Source: CAD feature listing. Evaluate the final solid. Frame: model axes, mm. A direction names the side the tool comes from. Give positions to 0.01 mm unless a question says otherwise; leave off trailing zeros. Order: outer loops, then holes, each group sorted by start corner. A loop starts at its lowest first (then second) coordinate and runs counter-clockwise, first axis right, second up. Notation, with made-up numbers: M 19,76 L 54,76 A28 cw 54,115 Z; hole C 48.25,83.5 d1. An arc over 180 degrees is marked long. Return JSON: item names as keys, results as strings.
from build123d import *

# Parameters (mm, degrees)
SKETCH_1_W          = 25
SKETCH_1_H          = 24
EXTRUDE_1_DEPTH     = 25
SKETCH_2_W          = 25
SKETCH_2_H          = 14.5
CUT_EXTRUDE_1_DEPTH = 5
SKETCH_3_R          = 1.5
CUT_EXTRUDE_2_DEPTH = 31.417922349
CUT_EXTRUDE_3_DEPTH = 37.84087404
SKETCH_6_R          = 3.5
CUT_EXTRUDE_4_DEPTH = 13
SKETCH_7_R          = 3.5
CUT_EXTRUDE_5_DEPTH = 7
SKETCH_8_R          = 1.25
CUT_EXTRUDE_6_DEPTH = 37.84087404


with BuildPart() as part:
    # 草图1 → 凸台-拉伸1 (new body)
    with BuildSketch(Plane(origin=(0, 0, 0), x_dir=(0, 0, -1), z_dir=(1, 0, 0))):
        Rectangle(SKETCH_1_W, SKETCH_1_H)
    extrude(amount=EXTRUDE_1_DEPTH)

    # 草图2 → 切除-拉伸1 (cut)
    with BuildSketch(Plane.ZY):
        Rectangle(SKETCH_2_W, SKETCH_2_H)
    extrude(amount=-CUT_EXTRUDE_1_DEPTH, mode=Mode.SUBTRACT)

    # 草图3 → 切除-拉伸2 (cut, through all)
    with BuildSketch(Plane(origin=(25, 0, 0), x_dir=(0, 0, -1), z_dir=(1, 0, 0))):
        with Locations((-2.5, 0)):
            Circle(SKETCH_3_R)
        with Locations((7.5, 0)):
            Circle(SKETCH_3_R)
    extrude(amount=-CUT_EXTRUDE_2_DEPTH, mode=Mode.SUBTRACT)

    # 草图5 → 切除-拉伸3 (cut, through all)
    with BuildSketch(Plane(origin=(0, 12, 0), x_dir=(1, 0, 0), z_dir=(0, 1, 0))):
        Polygon((12.5, 12.5), (25, -7.5), (25, 12.5), align=None)
    extrude(amount=-CUT_EXTRUDE_3_DEPTH, mode=Mode.SUBTRACT)

    # 草图6 → 切除-拉伸4 (cut)
    with BuildSketch(Plane(origin=(25, 0, 0), x_dir=(0, 0, -1), z_dir=(1, 0, 0))):
        with Locations((7.5, 0)):
            Circle(SKETCH_6_R)
    extrude(amount=-CUT_EXTRUDE_4_DEPTH, mode=Mode.SUBTRACT)

    # 草图7 → 切除-拉伸5 (cut)
    with BuildSketch(Plane(origin=(25, 0, 0), x_dir=(0, 0, -1), z_dir=(1, 0, 0))):
        with Locations((-2.5, 0)):
            Circle(SKETCH_7_R)
    extrude(amount=-CUT_EXTRUDE_5_DEPTH, mode=Mode.SUBTRACT)

    # 草图8 → 切除-拉伸6 (cut, through all)
    with BuildSketch(Plane(origin=(0, 12, 0), x_dir=(1, 0, 0), z_dir=(0, 1, 0))):
        with Locations(Location((12.5, 2.5, 0), (0, 0, 270))):
            Circle(SKETCH_8_R)
        with Locations(Location((12.5, -7.5, 0), (0, 0, 270))):
            Circle(SKETCH_8_R)
    extrude(amount=-CUT_EXTRUDE_6_DEPTH, mode=Mode.SUBTRACT)


solid = part.part
1. Section query B-B (y = 0). Return loops of the section in (x, z).
Evaluation:
{"outline": "M 5,-12.5 L 12.5,-12.5 L 13.44,-11 L 12,-11 L 12,-9 L 5,-9 Z; M 5,-6 L 12,-6 L 12,-4 L 17.81,-4 L 19.69,-1 L 18,-1 L 18,1 L 5,1 Z; M 5,4 L 18,4 L 18,6 L 24.06,6 L 25,7.5 L 25,12.5 L 5,12.5 Z; hole C 12.5,-2.5 d2.5; hole C 12.5,7.5 d2.5"}
2. Draft query along Y for faces 1 (the face through (13.345, 0.168, 6.579)), 2 (the face through (10, -12, 0)), 3 (the face through (20, 0, 6)), 4 (the face through (10, 12, 0)). Return one class per face: pulls with the +Y half, pulls with the -Y half, needs draft (parallel to the pull), parting line crosses it, or undercut.
Evaluation:
{"face 1": "needs draft", "face 2": "pulls with the -Y half", "face 3": "undercut", "face 4": "pulls with the +Y half"}
3. Section query C-C (x = 6.25). Return loops of the section in (y, z).
Evaluation:
{"outline": "M -12,-12.5 L 12,-12.5 L 12,12.5 L -12,12.5 Z; hole C 0,-7.5 d3; hole C 0,2.5 d3"}
4. Set-up query: faces 5 (the face through (5, 0, 0)), 6 (the face through (8, 0, -12.5)), 7 (the face through (14, 0, -4)). Return all of +Z, -Z, +X, -X, +Y, -Y with unobstructed straight access to the full face (end or side cutting, diameter ignored); none if empty.
Evaluation:
{"face 5": "+Z, -Z, -X", "face 6": "-Z, +X, -X, +Y, -Y", "face 7": "+X"}
5. Section query A-A (z = -2.5). Return loops of the section in (x, y), then the cut area to 4 significant figures.
Evaluation:
{"outline": "M 0,-12 L 11.25,-12 L 11.25,12 L 0,12 L 0,7.25 L 5,7.25 L 5,-7.25 L 0,-7.25 Z; M 13.75,-12 L 18.75,-12 L 18.75,12 L 13.75,12 Z", "area": "317.5 mm^2"}
6. Section query D-D (y = -6.5). Return loops of the section in (x, z).
Evaluation:
{"outline": "M 5,-12.5 L 12.5,-12.5 L 25,7.5 L 25,12.5 L 5,12.5 Z; hole C 12.5,-2.5 d2.5; hole C 12.5,7.5 d2.5"}
7. Ray query, probe 1 along Y at (x, z) = (8.25, -7.5); probe 2 along Z at (x, y) = (13, -1.75); probe 3 along Y at (x, z) = (15.25, -7.5). Return the intervals inside material, ascending.
Evaluation:
{"probe 1": "y = -12 to -1.5, 1.5 to 12", "probe 2": "z = -11.7 to -10.53, -4.47 to -3.65, -1.35 to 6.35, 8.65 to 12.5", "probe 3": "y = -12 to -3.5, 3.5 to 12"}
8. First-contact query: pin 1 (3 mm diameter, centred on y = 1.5, z = -1, fed in from -X); pin 2 (5.5 mm diameter, centred on y = 1.5, z = -7, fed in from +X); pin 3 (3 mm diameter, centred on x = 18, y = 5.5, fed in from -Z). Flat tips, straight axial feed; report the tip coordinate or a pass-through.
Evaluation:
{"pin 1": "stops at x = 5", "pin 2": "stops at x = 17.66", "pin 3": "stops at z = -6.1"}
